The listing builds one solid part. Answer for the finished solid, in the listing's coordinates (mm). Give positions to 0.01 mm unless a question says otherwise; leave off trailing zeros. Order: outer loops, then holes, each group sorted by start corner. A loop starts at its lowest first (then second) coordinate and runs counter-clockwise, first axis right, second up.
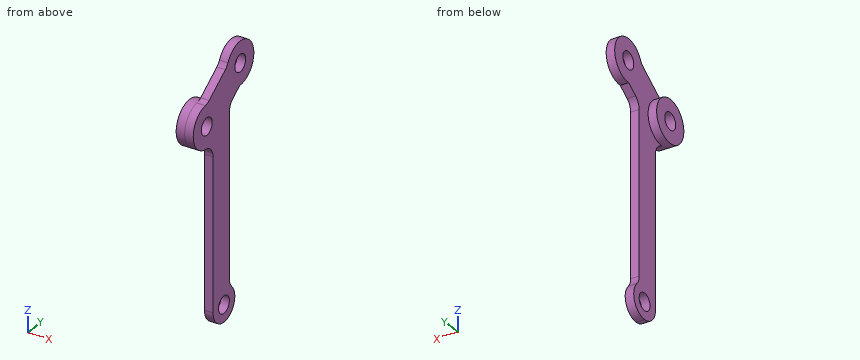
```python
from build123d import *

# Parameters (mm, degrees)
EXTRUDE_1_DEPTH          = 2
EXTRUDE_START            = -2
SKETCH_1_4_R             = 5
EXTRUDE_2_DEPTH          = 2
CUT_EXTRUDE_1_DEPTH      = 51.040969284
CUT_EXTRUDE_1_DEPTH_BACK = 51.040969284
SKETCH_1_3_R             = 2
FILLET_1_R               = 3


with BuildPart() as part:
    # 草图1 → 凸台-拉伸1 (new body)
    with BuildSketch(Plane(origin=(0, 0, 0), x_dir=(0, 0, -1), z_dir=(1, 0, 0))):
        with BuildLine():
            Line((40.737143614, 0), (0, 0))
            Line((0, 0), (2.48051592, -3.542543867))
            ThreePointArc((2.48051592, -3.542543867), (4.165783411, -4.487079684), (5.367176995, -6))
            Line((5.367176995, -6), (44.201245229, -6))
            ThreePointArc((44.201245229, -6), (40.737143614, -4), (40.737143614, 0))
        make_face()
        with BuildLine():
            Line((2.48051592, -3.542543867), (0, 0))
            Line((0, 0), (-2.681672007, 3.829824531))
            ThreePointArc((-2.681672007, 3.829824531), (-4.811127311, -0.102785303), (-9.234888361, -0.758786959))
            Line((-9.234888361, -0.758786959), (-4.072700434, -8.131155358))
            ThreePointArc((-4.072700434, -8.131155358), (-1.94324513, -4.198545524), (2.48051592, -3.542543867))
        make_face()
        with BuildLine():
            ThreePointArc((48.201245229, -2), (45.23652141, 1.863703305), (40.737143614, 0))
            Line((40.737143614, 0), (44.201245229, 0))
            ThreePointArc((44.201245229, 0), (45.615458792, -0.585786438), (46.201245229, -2))
            ThreePointArc((46.201245229, -2), (45.615458792, -3.414213562), (44.201245229, -4))
            Line((44.201245229, -4), (44.201245229, -6))
            ThreePointArc((44.201245229, -6), (47.029672354, -4.828427125), (48.201245229, -2))
        make_face()
        with BuildLine():
            Line((44.201245229, 0), (40.737143614, 0))
            ThreePointArc((40.737143614, 0), (40.737143614, -4), (44.201245229, -6))
            Line((44.201245229, -6), (44.201245229, -4))
            ThreePointArc((44.201245229, -4), (42.201245229, -2), (44.201245229, 0))
        make_face()
        with BuildLine():
            ThreePointArc((5.367176995, -6), (4.165783411, -4.487079684), (2.48051592, -3.542543867))
            Line((2.48051592, -3.542543867), (4.201245229, -6))
            Line((4.201245229, -6), (5.367176995, -6))
        make_face()
        with BuildLine():
            Line((4.201245229, -6), (2.48051592, -3.542543867))
            ThreePointArc((2.48051592, -3.542543867), (-1.94324513, -4.198545524), (-4.072700434, -8.131155358))
            Line((-4.072700434, -8.131155358), (-2.351971125, -10.588611491))
            Line((-2.351971125, -10.588611491), (-0.713667036, -9.441458618))
            ThreePointArc((-0.713667036, -9.441458618), (-0.222515821, -6.656001657), (2.562941141, -7.147152873))
            Line((2.562941141, -7.147152873), (4.201245229, -6))
        make_face()
        with BuildLine():
            ThreePointArc((-9.234888361, -0.758786959), (-4.811127311, -0.102785303), (-2.681672007, 3.829824531))
            Line((-2.681672007, 3.829824531), (-4.402401316, 6.287280664))
            Line((-4.402401316, 6.287280664), (-6.040705405, 5.140127792))
            ThreePointArc((-6.040705405, 5.140127792), (-5.771575592, 4.594386518), (-5.679009493, 3.992974919))
            ThreePointArc((-5.679009493, 3.992974919), (-7.077597894, 2.085541017), (-9.317313582, 2.845822046))
            Line((-9.317313582, 2.845822046), (-10.95561767, 1.698669174))
            Line((-10.95561767, 1.698669174), (-9.234888361, -0.758786959))
        make_face()
        with BuildLine():
            Line((-4.402401316, 6.287280664), (-2.681672007, 3.829824531))
            ThreePointArc((-2.681672007, 3.829824531), (-2.679675166, 3.911388863), (-2.679009493, 3.992974919))
            ThreePointArc((-2.679009493, 3.992974919), (-10.613341245, 8.041394014), (-9.234888361, -0.758786959))
            Line((-9.234888361, -0.758786959), (-10.95561767, 1.698669174))
            Line((-10.95561767, 1.698669174), (-9.317313582, 2.845822046))
            ThreePointArc((-9.317313582, 2.845822046), (-8.826162366, 5.631279008), (-6.040705405, 5.140127792))
            Line((-6.040705405, 5.140127792), (-4.402401316, 6.287280664))
        make_face()
        with BuildLine():
            ThreePointArc((46.201245229, -2), (45.615458792, -0.585786438), (44.201245229, 0))
            Line((44.201245229, 0), (44.201245229, -4))
            ThreePointArc((44.201245229, -4), (45.615458792, -3.414213562), (46.201245229, -2))
        make_face()
        with BuildLine():
            Line((44.201245229, -4), (44.201245229, 0))
            ThreePointArc((44.201245229, 0), (42.201245229, -2), (44.201245229, -4))
        make_face()
        with BuildLine():
            Line((5.367176995, -6), (4.201245229, -6))
            Line((4.201245229, -6), (2.562941141, -7.147152873))
            ThreePointArc((2.562941141, -7.147152873), (2.832070954, -7.692894146), (2.924637052, -8.294305745))
            ThreePointArc((2.924637052, -8.294305745), (1.526048651, -10.201739647), (-0.713667036, -9.441458618))
            Line((-0.713667036, -9.441458618), (-2.351971125, -10.588611491))
            Line((-2.351971125, -10.588611491), (-4.072700434, -8.131155358))
            ThreePointArc((-4.072700434, -8.131155358), (0.843050996, -13.293640073), (5.924637052, -8.294305745))
            ThreePointArc((5.924637052, -8.294305745), (5.783273678, -7.113776143), (5.367176995, -6))
        make_face()
        with BuildLine():
            ThreePointArc((2.924637052, -8.294305745), (2.832070954, -7.692894146), (2.562941141, -7.147152873))
            Line((2.562941141, -7.147152873), (-0.713667036, -9.441458618))
            ThreePointArc((-0.713667036, -9.441458618), (1.526048651, -10.201739647), (2.924637052, -8.294305745))
        make_face()
        with BuildLine():
            Line((-0.713667036, -9.441458618), (2.562941141, -7.147152873))
            ThreePointArc((2.562941141, -7.147152873), (-0.222515821, -6.656001657), (-0.713667036, -9.441458618))
        make_face()
        with BuildLine():
            ThreePointArc((-5.679009493, 3.992974919), (-5.771575592, 4.594386518), (-6.040705405, 5.140127792))
            Line((-6.040705405, 5.140127792), (-9.317313582, 2.845822046))
            ThreePointArc((-9.317313582, 2.845822046), (-7.077597894, 2.085541017), (-5.679009493, 3.992974919))
        make_face()
        with BuildLine():
            Line((-9.317313582, 2.845822046), (-6.040705405, 5.140127792))
            ThreePointArc((-6.040705405, 5.140127792), (-8.826162366, 5.631279008), (-9.317313582, 2.845822046))
        make_face()
    extrude(amount=EXTRUDE_1_DEPTH)

    # 草图1<4> → 凸台-拉伸2 (add)
    with BuildSketch(Plane(origin=(0, 0, 0), x_dir=(0, 0, -1), z_dir=(1, 0, 0)).offset(EXTRUDE_START)):
        with Locations(Location((0.924637052, -8.294305745, 0), (0, 0, 178.130102354))):
            Circle(SKETCH_1_4_R)
    extrude(amount=EXTRUDE_2_DEPTH)

    # 草图1<3> → 切除-拉伸1 (cut, two sides: drawn at the far end of the back side and taken through both)
    with BuildSketch(Plane(origin=(0, 0, 0), x_dir=(0, 0, -1), z_dir=(1, 0, 0)).offset(-CUT_EXTRUDE_1_DEPTH_BACK)):
        with Locations((-7.679009493, 3.992974919)):
            Circle(SKETCH_1_3_R)
        with Locations((44.201245229, -2)):
            Circle(SKETCH_1_3_R)
        with Locations((0.924637052, -8.294305745)):
            Circle(SKETCH_1_3_R)
    extrude(amount=CUT_EXTRUDE_1_DEPTH + CUT_EXTRUDE_1_DEPTH_BACK, mode=Mode.SUBTRACT)

    # 圆角1
    # the kernel refuses this fillet: 3 mm, written as the material it adds along each edge
    with BuildSketch(Plane(origin=(0, -6, -5.367176995), x_dir=(0, 0, -1), z_dir=(1, 0, 0))) as fillet_1_piece_1:
        with BuildLine():
            CenterArc((3.526273997, -3), FILLET_1_R, 90, 84.939259464)
            ThreePointArc((0.53796877, -2.735364655), (0.463478447, -1.329430853), (0, 0))
            Line((0, 0), (3.526273997, 0))
        make_face()
    extrude(amount=2)
    with BuildSketch(Plane(origin=(0, 0, 0), x_dir=(0, 0, -1), z_dir=(1, 0, 0))) as fillet_1_piece_2:
        with BuildLine():
            CenterArc((FILLET_1_R * 0.520567050552, FILLET_1_R), FILLET_1_R, 215, 55)
            Line((-FILLET_1_R * 0.298584993737, FILLET_1_R * 0.426423563649), (0, 0))
            Line((0, 0), (FILLET_1_R * 0.520567050552, 0))
        make_face()
    extrude(amount=2)
    with BuildSketch(Plane(origin=(0, 0, -40.737143614), x_dir=(0, 0.790236885240252, -0.6128014892326752), z_dir=(1, 0, 0))) as fillet_1_piece_3:
        with BuildLine():
            CenterArc((1.49141536, 2.972297887), FILLET_1_R, 217.792345701, 44.415308597)
            Line((-0.879295296, 1.133893419), (0, 0))
            ThreePointArc((0, 0), (0.542332858, 0.036936151), (1.084665716, 0))
        make_face()
    extrude(amount=2)
    with BuildSketch(Plane(origin=(0, -0.758786959, 9.234888361), x_dir=(0, -0.8191520442889745, -0.5735764363510707), z_dir=(1, 0, 0))) as fillet_1_piece_4:
        with BuildLine():
            CenterArc((0.872983346, -3), FILLET_1_R, 90, 28.955024372)
            ThreePointArc((-0.579385409, -0.375), (-0.283214788, -0.19750856), (0, 0))
            Line((0, 0), (0.872983346, 0))
        make_face()
    extrude(amount=2)
    with BuildSketch(Plane(origin=(0, -8.131155358, 4.072700434), x_dir=(0, -0.9993363396246481, -0.03642636827368134), z_dir=(1, 0, 0))) as fillet_1_piece_5:
        with BuildLine():
            CenterArc((0.897200113, -2.992846785), FILLET_1_R, 93.957436637, 28.955024372)
            Line((-0.732871014, -0.474341649), (0, 0))
            ThreePointArc((0, 0), (0.345076967, -0.011922025), (0.690153933, 0))
        make_face()
    extrude(amount=2)


solid = part.part
```
1) Find section A-A (x = 1.2). Write down the section's boundary in (y, z).
Geometry says:
outline: (-8.82, 4.05) arc R5 ccw to (-8.74, -5.91) arc R3 cw to (-6, -8.89) - (-6, -44.2) arc R4 ccw (long way) to (0.86, -41.4) arc R3 cw to (0, -39.3) - (0, -1.56) arc R3 cw to (1.28, 0.9) - (3.83, 2.68) arc R5 ccw to (3.99, 2.68) arc R5 ccw (long way) to (-0.5, 9.87) arc R3 cw to (-1.47, 8.73) - (-7.42, 4.57) arc R3 cw to start; hole circle Ø4 at (-8.29, -0.92); hole circle Ø4 at (-2, -44.2); hole circle Ø4 at (3.99, 7.68)
2) Straight lines are drawn through the part: probe 1 along Y at (x, z) = (0.5, 0); probe 2 along X at (y, z) = (-5.75, -7.5); probe 3 along Y at (x, z) = (1.5, -30.5). For each, find the intervals that lie inside material, in ascending order.
Geometry says:
probe 1: y = -13.21 to -10.07, -6.52 to 0.44
probe 2: x = 0 to 2
probe 3: y = -6 to 0
3) Given P1, Ø2, axis at x = 1, z = -19, coming from the -Y side; P2, Ø6.5, axis at y = -2, z = -44.2, coming from the -X side; P3, Ø1, axis at x = 1, z = -15.5, coming from the +Y side, each flat-ended and moving along its own axis, determine where each tip first touches the part or whether it passes through.
Geometry says:
P1: stops at y = -6
P2: stops at x = 0
P3: stops at y = 0
4) Find section B-B (z = -22.5). Write down the section's boundary in (x, y), then the cut area to 3 significant figures.
Geometry says:
outline: (0, -6) - (2, -6) - (2, 0) - (0, 0) - close
area: 12.0 mm2
